Work out the finished part from the listing and answer in its coordinate system (mm). Face numbers are marked on the shaded views. A direction names the side the tool comes from. Round coordinates to 2 decimals unless told otherwise and drop trailing zeros. Loops run counter-clockwise (first coordinate to the right, second up) from the corner with the lowest first, then second, coordinate; pieces in that order, holes last.
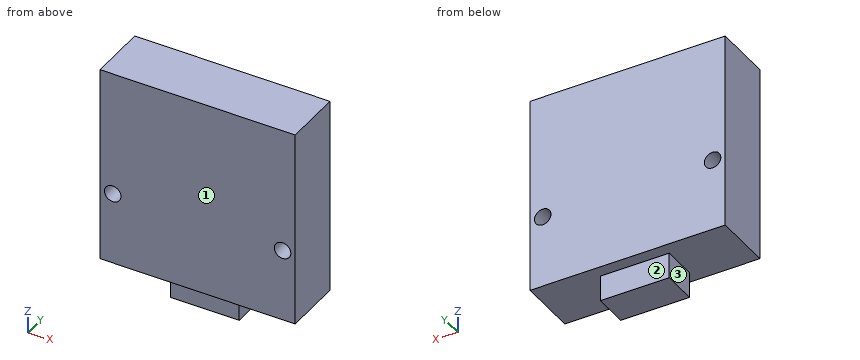
```python
from build123d import *

# Parameters (mm, degrees)
SKETCH1_W                        = 117.475
SKETCH1_H                        = 35.56
EXTRUDE1_DEPTH                   = 119.38
SKETCH2_W                        = 41.402
SKETCH2_H                        = 20.828
EXTRUDE2_DEPTH                   = 15.494
F_25_64_0_39063_DIAMETER_HOLE1_D = 9.922002


with BuildPart() as part:
    # Sketch1 → Extrude1 (new body)
    with BuildSketch(Plane.XY):
        Rectangle(SKETCH1_W, SKETCH1_H)
    extrude(amount=EXTRUDE1_DEPTH)

    # Sketch2 → Extrude2 (add)
    with BuildSketch(Plane(origin=(0, 0, 0), x_dir=(-1, 0, 0), z_dir=(0, 0, -1))):
        Rectangle(SKETCH2_W, SKETCH2_H)
    extrude(amount=EXTRUDE2_DEPTH)

    # 25/64 (0.39063) Diameter Hole1 (through all)
    with Locations(Plane(origin=(-51.1175, -17.78, 43.688), x_dir=(0, 0, -1), z_dir=(0, -1, 0))):
        with Locations((0, 0), (0, 102.235)):
            Hole(F_25_64_0_39063_DIAMETER_HOLE1_D / 2)


solid = part.part
```
1. Find section A-A (z = 43). Write down the section's boundary in (x, y).
Answer key:
outline: (-58.74, -17.78) - (-56.03, -17.78) - (-56.03, 17.78) - (-58.74, 17.78) - close; (-46.2, -17.78) - (46.2, -17.78) - (46.2, 17.78) - (-46.2, 17.78) - close; (56.03, -17.78) - (58.74, -17.78) - (58.74, 17.78) - (56.03, 17.78) - close
2. Find section C-C (y = 7). Write down the section's boundary in (x, z), then the cut area to 3 significant figures.
Answer key:
outline: (-58.74, 0) - (-20.7, 0) - (-20.7, -15.49) - (20.7, -15.49) - (20.7, 0) - (58.74, 0) - (58.74, 119.38) - (-58.74, 119.38) - close; hole circle Ø9.92 at (-51.12, 43.69); hole circle Ø9.92 at (51.12, 43.69)
area: 14,500 mm2
3. Find section D-D (x = -25). Write down the section's boundary in (y, z).
Answer key:
outline: (-17.78, 0) - (17.78, 0) - (17.78, 119.38) - (-17.78, 119.38) - close
4. Consider probe 1 along Z at (x, y) = (44.5, 11.5); probe 2 along X at (y, z) = (0, -4); probe 3 along Z at (x, y) = (-48, -8.5). Determine where each line is inside the solid, lowest interval first.
Answer key:
probe 1: z = 0 to 119.38
probe 2: x = -20.7 to 20.7
probe 3: z = 0 to 39.83, 47.55 to 119.38
5. Given pin 1 (3 mm diameter, centred on x = -26.5, y = 11, fed in from -Z); pin 2 (17 mm diameter, centred on y = -2.5, z = -9.5, fed in from -X); pin 3 (9 mm diameter, centred on x = -51.12, z = 43.69, fed in from +Y); pin 4 (4.5 mm diameter, centred on x = -8.5, z = -5, fed in from -Y), each flat-ended and moving along its own axis, determine where each tip first touches the part or whether it passes through.
Answer key:
pin 1: stops at z = 0
pin 2: stops at x = -20.7
pin 3: passes through
pin 4: stops at y = -10.41
6. Find section B-B (x = -6). Write down the section's boundary in (y, z), then the cut area to 3 significant figures.
Answer key:
outline: (-17.78, 0) - (-10.41, 0) - (-10.41, -15.49) - (10.41, -15.49) - (10.41, 0) - (17.78, 0) - (17.78, 119.38) - (-17.78, 119.38) - close
area: 4,570 mm2
7. Which of the six approach directions +Z, -Z, +X, -X, +Y, -Y give full straight-line access (tool end or side, diameter ignored) to the marked faces 1, 2 and 3?
Answer key:
face 1: +Z, -Z, +X, -X, -Y
face 2: -Z, +X, -X, +Y
face 3: -Z, -X, +Y, -Y
